Read the model definition and answer for the solid it produces. Units are mm, in the model's axes. A direction names the side the tool comes from. Give positions to 0.01 mm unless a question says otherwise; leave off trailing zeros. Loops run counter-clockwise (first coordinate to the right, second up) from the corner with the lowest first, then second, coordinate; pieces in that order, holes last. Notation, with made-up numbers: (82, 58.25) - (119, 58.25) arc R13 cw to (119, 63.25) - close; hole circle Ø5 at (49, 4). An arc over 180 degrees is marked (long way). Use a Markdown table: item, result. Add a question column.
Item 1: Which of the six approach directions +Z, -Z, +X, -X, +Y, -Y give full straight-line access (tool end or side, diameter ignored) to faces 1 (the face through (0, 25.567, 14)), 2 (the face through (74, 4, 14)), 3 (the face through (4, 28, 14))?
Item 2: Each of these flat-tipped pins is pushed along its axis until it touches: P1, Ø2, axis at x = 7.5, z = 13.5, coming from the +Y side; P2, Ø1.5, axis at x = 32.5, z = 15.5, coming from the +Y side; P3, Ø1.5, axis at y = -26.5, z = 13, coming from the +X side. Where does it stop, or does it pass through?
Item 3: A cutting plane is placed at C-C (y = -12). Determine the outline of the cut face in (x, z).
Item 4: For a pull along Y with two mould halves and no side action, classify faces 4 (the face through (39, 0, 17.35)), 5 (the face through (74, -4, 14)), 6 (the face through (0, -25.567, 14)), 7 (the face through (17.52, 30.213, 14.131)) as +Y half, -Y half, draft (parallel to the pull), parting line (faces both ways), or undercut.
Item 5: Consider probe 1 along Y at (x, z) = (56.5, 13.25); probe 2 along X at (y, z) = (1, 11.5); probe 3 along Y at (x, z) = (8.5, 14.5). Determine where each line is inside the solid, lowest interval first. Write a range as [from, to].
Item 6: A cutting plane is placed at B-B (x = 70). Determine the outline of the cut face in (y, z), plus the area to 3 significant figures.
from build123d import *

# Parameters (mm, degrees)
F0_R     = 18.25
F1_DEPTH = 11
F3_DEPTH = 6.35
F4_R     = 3.175
F5_R     = 0.79375


with BuildPart() as f1:
    # F0 (on Top) → F1 (new body)
    with BuildSketch(Plane.XY):
        with BuildLine():
            Line((-24.7792251695, -4), (-28.6218448043, -4))
            ThreePointArc((-28.6218448043, -4), (-20.4353859763, -20.4353859763), (-4, -28.6218448043))
            Line((-4, -28.6218448043), (-4, -24.7792251695))
            ThreePointArc((-4, -24.7792251695), (0, -25.1), (4, -24.7792251695))
            Line((4, -24.7792251695), (4, -28.6218448043))
            ThreePointArc((4, -28.6218448043), (20.4353859763, -20.4353859763), (28.6218448043, -4))
            Line((28.6218448043, -4), (24.7792251695, -4))
            ThreePointArc((24.7792251695, -4), (25.1, 0), (24.7792251695, 4))
            Line((24.7792251695, 4), (28.6218448043, 4))
            ThreePointArc((28.6218448043, 4), (20.4353859763, 20.4353859763), (4, 28.6218448043))
            Line((4, 28.6218448043), (4, 24.7792251695))
            ThreePointArc((4, 24.7792251695), (0, 25.1), (-4, 24.7792251695))
            Line((-4, 24.7792251695), (-4, 28.6218448043))
            ThreePointArc((-4, 28.6218448043), (-20.4353859763, 20.4353859763), (-28.6218448043, 4))
            Line((-28.6218448043, 4), (-24.7792251695, 4))
            ThreePointArc((-24.7792251695, 4), (-25.1, 0), (-24.7792251695, -4))
        make_face()
        Circle(F0_R, mode=Mode.SUBTRACT)
    extrude(amount=F1_DEPTH)


with BuildPart() as f3:
    # F2 (on face) → F3 (new body)
    with BuildSketch(Plane.XY.offset(11)):
        with BuildLine():
            Line((-4, -28.6218448043), (-4, -34.6951815819))
            ThreePointArc((-4, -34.6951815819), (15.925151873, -31.0828757167), (30.4965472195, -17.0210526316))
            ThreePointArc((30.4965472195, -17.0210526316), (39.8163298639, -7.4958307261), (52.6758542883, -4))
            Line((52.6758542883, -4), (98.1951815819, -4))
            Line((98.1951815819, -4), (98.1951815819, 4))
            Line((98.1951815819, 4), (52.6758542883, 4))
            ThreePointArc((52.6758542883, 4), (39.8163298639, 7.4958307261), (30.4965472195, 17.0210526316))
            ThreePointArc((30.4965472195, 17.0210526316), (15.925151873, 31.0828757167), (-4, 34.6951815819))
            Line((-4, 34.6951815819), (-4, 28.6218448043))
            Line((-4, 28.6218448043), (-4, 25.5670565819))
            Line((-4, 25.5670565819), (4, 25.5670565819))
            Line((4, 25.5670565819), (4, 28.6218448043))
            Line((4, 28.6218448043), (4, 29.7321374946))
            ThreePointArc((4, 29.7321374946), (30, 0), (4, -29.7321374946))
            Line((4, -29.7321374946), (4, -28.6218448043))
            Line((4, -28.6218448043), (4, -25.5670565819))
            Line((4, -25.5670565819), (-4, -25.5670565819))
            Line((-4, -25.5670565819), (-4, -28.6218448043))
        make_face()
    extrude(amount=F3_DEPTH)

    # F4
    f4_edges = [f3.edges().sort_by_distance(p)[0] for p in [
        (-4, -34.695182, 14.175),
        (-4, 34.695182, 14.175),
        (98.195182, -4, 14.175),
        (98.195182, 4, 14.175),
    ]]
    fillet(f4_edges, radius=F4_R)

    # F5
    f5_edges = [f3.edges().sort_by_distance(p)[0] for p in [
        (-4, -25.567057, 14.175),
        (4, -25.567057, 14.175),
        (-4, 25.567057, 14.175),
        (4, 25.567057, 14.175),
    ]]
    fillet(f5_edges, radius=F5_R)


solid = f3.part
Geometry says:
| question | item | result |
|---|---|---|
| 1 | face 1 | +Z, -Z, -X |
| 1 | face 2 | +Z, -Z, +X, +Y |
| 1 | face 3 | +Z, -Z |
| 2 | P1 | y = 34.31 |
| 2 | P2 | y = 15 |
| 2 | P3 | x = 23.59 |
| 3 | outline | (27.5, 11) - (34.17, 11) - (34.17, 17.35) - (27.5, 17.35) - close |
| 4 | face 4 | draft |
| 4 | face 5 | -Y half |
| 4 | face 6 | undercut |
| 4 | face 7 | +Y half |
| 5 | probe 1 | [-4, 4] |
| 5 | probe 2 | [29.98, 98.19] |
| 5 | probe 3 | [-33.87, -28.77], [28.77, 33.87] |
| 6 | outline | (-4, 11) - (4, 11) - (4, 17.35) - (-4, 17.35) - close |
| 6 | area | 50.8 mm² |
